Could you check a few things on this model? Use its own coordinates, in mm. A direction names the side the tool comes from. Round coordinates to 2 decimals unless told otherwise and drop trailing zeros. Loops run counter-clockwise (first coordinate to the right, second up) from the corner with the lowest first, then second, coordinate; pieces in that order, holes last.
Autodesk Inventor part; units mm, degrees
ref_plane "YZ Plane" through (0, 0, 0) normal (1, 0, 0) x (0, 1, 0)
ref_plane "XZ Plane" through (0, 0, 0) normal (0, 1, 0) x (-1, 0, 0)
ref_plane "XY Plane" through (0, 0, 0) normal (0, 0, 1) x (1, 0, 0)
sketch "Sketch1" plane through (0, 0, 0) normal (0, 0, 1) x (1, 0, 0)
  line L0 (-16, 12.5) -> (-13, 12.5)
  line L1 (-13, 12.5) -> (-13, -9.5)
  line L2 (-13, -9.5) -> (13, -9.5)
  line L3 (13, -9.5) -> (13, 12.9)
  line L4 (13, 12.9) -> (16, 12.9)
  line L5 (16, 12.9) -> (16, -12.5)
  line L6 (16, -12.5) -> (-16, -12.5)
  line L7 (-16, -12.5) -> (-16, 12.5)
  point P0 (0, 0)
  dimension "d0" = 3
  dimension "d2" = 3
  dimension "d3" = 25
  dimension "d4" = 32
  dimension "d5" = 16
  dimension "d7" = 12.5
  dimension "d8" = 3
extrude "Extrusion1" add sketch "Sketch1" against normal blind 482.6
sketch "Sketch4" plane through (16, -12.5, 0) normal (1, 0, 0) x (0, 0, -1)
  line L0 (0, 25.4) -> (0, 0)
  line L1 (482.6, 25.4) -> (482.6, 0)
  line L2 (0, 25.4) -> (482.6, 25.4)
  circle A0 centre (12.7, 12.7) radius 3.175
  circle A1 centre (469.9, 12.7) radius 3.175
  point P0 (0, 12.5)
  dimension "d21" = 6.35
  dimension "d24" = 12.7
  dimension "d26" = 12.7
  dimension "d27" = 6.35
  dimension "d28" = 12.7
  dimension "d29" = 12.7
hole "Mount Hole" at (16, 0.2, -12.7) at (16, 0.2, -469.9) direction (-1, 0, 0) diameter 6.35 depth 12.7 tip angle 118
sketch "Sketch5" plane through (-16, -12.5, 0) normal (-1, 0, 0) x (0, 0, 1)
  circle A0 centre (-12.7, 12.7) radius 3.175
  circle A1 centre (-469.9, 12.7) radius 3.175
  circle A2 centre (-469.9, 12.7) radius 4.7625
  circle A3 centre (-12.7, 12.7) radius 4.7625
  point P0 (0, 12.5)
  dimension "d37" = 9.525
  dimension "d38" = 9.525
hole "Access Hole" at (-16, 0.2, -469.9) at (-16, 0.2, -12.7) direction (1, 0, 0) diameter 9.525 depth 3 tip angle 118
sketch "Sketch6" plane through (-16, -12.5, 0) normal (-1, 0, 0) x (0, 0, 1)
  line L0 (0, 0) -> (0, 25)
  line L1 (-482.6, 0) -> (-482.6, 25)
  line L2 (0, 0) -> (-482.6, 0)
  circle A0 centre (-431.519, 15.5) radius 3.175
  circle A1 centre (-51.081, 15.5) radius 3.175
  point P0 (0, 12.5)
  dimension "d46" = 6.35
  dimension "d47" = 51.081
  dimension "d48" = 15.5
  dimension "d49" = 6.35
  dimension "d50" = 51.081
hole "Hole3" at (-16, 3, -431.519) at (-16, 3, -51.081) direction (1, 0, 0) diameter 6.35 depth 3 tip angle 118
equation "\"d2\" = d0"
equation "\"d8\" = d0"
equation "\"d24\" = d26"
equation "\"d27\" = d21"
equation "\"d28\" = d26"
equation "\"d29\" = d24"
equation "\"d35\" = d24"
equation "\"d38\" = d37"
equation "\"d50\" = d47"
properties part number "Rack - Back"
Item 1: We'd pull the mould along Y, two halves only. Please class faces 4 (the cylindrical face through (-14.479, -1.231, -8.157)), 5 (the flat face through (0, -12.5, -238)), 6 (the flat face through (-1, -10, 0)): released by +Y, released by -Y, zero draft, split by the parting line, or undercut.
Results list:
face 4: undercut
face 5: released by -Y
face 6: zero draft
Item 2: For faces 1 (the cylindrical face through (-14.479, -1.231, -465.357)), 2 (the flat face through (16, 0, -238)), 3 (the flat face through (-13, 2, -238)), which set-ups out of +Z, -Z, +X, -X, +Y, -Y let a thin tool reach every point of the face, with its end or its side?
Results list:
face 1: -X
face 2: +Z, -Z, +X, +Y, -Y
face 3: +Z, -Z, +Y
Item 3: If we section it at B-B, the plane x = -2.5: Please give me the cut outline in (y, z).
Results list:
outline: (-12.5, -482.6) - (-9.5, -482.6) - (-9.5, 0) - (-12.5, 0) - close
Item 4: If I drill on line 1 along Z through (x, y) = (14.65, 0.2) (3 decimals); line 2 along X through (y, z) = (-9, -290); line 3 along Z through (x, y) = (-14.7, 3), over which ranges is the centre line in solid material (lowest first)?
Results list:
line 1: z = -482.6 to -473.075, -466.725 to -15.875, -9.525 to 0
line 2: x = -16 to -13, 13 to 16
line 3: z = -482.6 to -473.75, -466.05 to -434.69, -428.34 to -54.26, -47.91 to -16.55, -8.85 to 0
Item 5: Will these pins go through, and if not, where does the flat tip stop? pin 1 (7.5 mm diameter, centred on y = 0.2, z = -469.9, fed in from -X); pin 2 (12.5 mm diameter, centred on y = 0.2, z = -469.9, fed in from -X); pin 3 (8 mm diameter, centred on x = -4, z = -342, fed in from +Y); pin 4 (1.5 mm diameter, centred on x = -15, z = -247, fed in from +Y).
Results list:
pin 1: stops at x = 13
pin 2: stops at x = -16
pin 3: stops at y = -9.5
pin 4: stops at y = 12.5
Item 6: If we section it at A-A, the plane z = -282: Please give me the cut outline in (x, y).
Results list:
outline: (-16, -12.5) - (16, -12.5) - (16, 12.9) - (13, 12.9) - (13, -9.5) - (-13, -9.5) - (-13, 12.5) - (-16, 12.5) - close
